```python
from build123d import *

# Parameters (mm, degrees)
SALIENTE_EXTRUIR1_DEPTH = 30
CROQUIS2_R              = 2.5
CORTAR_EXTRUIR1_DEPTH   = 71.10083252
CROQUIS3_W              = 27
CROQUIS3_H              = 62.627315121
CORTAR_EXTRUIR2_DEPTH   = 72
CORTAR_EXTRUIR3_DEPTH   = 64.283609709


with BuildPart() as part:
    # Croquis1 → Saliente-Extruir1 (new body)
    with BuildSketch(Plane.XY):
        with BuildLine():
            Line((-13.910195184, 10.658823529), (-13.910195184, 39.47248109))
            ThreePointArc((-13.910195184, 39.47248109), (-12.082079753, 42.831486511), (-8.268736475, 43.12016711))
            Line((-8.268736475, 43.12016711), (46.089804816, 18.658823529))
            Line((46.089804816, 18.658823529), (46.089804816, 10.658823529))
            Line((46.089804816, 10.658823529), (-13.910195184, 10.658823529))
        make_face()
    extrude(amount=SALIENTE_EXTRUIR1_DEPTH)

    # Croquis2 → Cortar-Extruir1 (cut, through all)
    with BuildSketch(Plane.XY.offset(30)):
        with Locations((-9.910195184, 39.47248109)):
            Circle(CROQUIS2_R)
    extrude(amount=-CORTAR_EXTRUIR1_DEPTH, mode=Mode.SUBTRACT)

    # Croquis3 → Cortar-Extruir2 (cut)
    with BuildSketch(Plane.ZY.offset(13.910195184)):
        with Locations((15, 43.47248109)):
            Rectangle(CROQUIS3_W, CROQUIS3_H)
    extrude(amount=-CORTAR_EXTRUIR2_DEPTH, mode=Mode.SUBTRACT)

    # Croquis4 → Cortar-Extruir3 (cut, through all)
    with BuildSketch(Plane(origin=(0, 12.158823529, 0), x_dir=(1, 0, 0), z_dir=(0, 1, 0))):
        with BuildLine():
            Line((-33.910195184, -20), (6.089804816, -20))
            ThreePointArc((6.089804816, -20), (11.089804816, -15), (6.089804816, -10))
            Line((6.089804816, -10), (-33.910195184, -10))
            Line((-33.910195184, -10), (-33.910195184, -20))
        make_face()
    extrude(amount=-CORTAR_EXTRUIR3_DEPTH, mode=Mode.SUBTRACT)


solid = part.part
```
Geometry: final body of the model. Coordinates: model frame, mm. A direction names the side the tool comes from. Round coordinates to 2 decimals unless told otherwise and drop trailing zeros. Loops run counter-clockwise (first coordinate to the right, second up) from the corner with the lowest first, then second, coordinate; pieces in that order, holes last. Notation, with made-up numbers: (35, -16) -> (83, -16) arc R17 cw to (83, 16) -> close; hole circle Ø10 at (65.5, 28.5). An arc over 180 degrees is marked (long way). Use one line per item in the form item = value.
Item 1: Material intervals for probe 1 along Z at (x, y) = (41, 14); probe 2 along Y at (x, z) = (31, 21.25), sorted ascending.
Evaluation:
probe_1 = 0 to 1.5, 28.5 to 30
probe_2 = 10.66 to 12.16
Item 2: Cut plane C-C on y = 38. Output: boundary loops of the cut face in (x, z), then the cut area to 3 significant figures.
Evaluation:
outline = (-13.91, 0) -> (-11.93, 0) -> (-11.93, 1.5) -> (-13.91, 1.5) -> close; (-13.91, 28.5) -> (-11.93, 28.5) -> (-11.93, 30) -> (-13.91, 30) -> close; (-7.89, 0) -> (3.11, 0) -> (3.11, 1.5) -> (-7.89, 1.5) -> close; (-7.89, 28.5) -> (3.11, 28.5) -> (3.11, 30) -> (-7.89, 30) -> close
area = 38.9 mm2
Item 3: Cut plane A-A on y = 17.5. Output: boundary loops of the cut face in (x, z), then the cut area to 3 significant figures.
Evaluation:
outline = (-13.91, 0) -> (46.09, 0) -> (46.09, 1.5) -> (-13.91, 1.5) -> close; (-13.91, 28.5) -> (46.09, 28.5) -> (46.09, 30) -> (-13.91, 30) -> close
area = 180 mm2
Item 4: Draft query along X for faces 4 (the cylindrical face through (11.09, 11.42, 15.11)), 5 (the cylindrical face through (-11.753, 41.162, 29.26)), 6 (the flat face through (46.09, 12, 18)), 7 (the cylindrical face through (-11.753, 41.162, 0.761)). Return one class per face: released by +X, released by -X, zero draft, split by the parting line, or undercut.
Evaluation:
face_4 = released by -X
face_5 = undercut
face_6 = released by +X
face_7 = undercut
Item 5: Cut plane D-D on x = 37. Output: boundary loops of the cut face in (y, z).
Evaluation:
outline = (10.66, 0) -> (22.75, 0) -> (22.75, 1.5) -> (12.16, 1.5) -> (12.16, 28.5) -> (22.75, 28.5) -> (22.75, 30) -> (10.66, 30) -> close
Item 6: Access query for faces 1 (the flat face through (-4, 11, 10)), 2 (the flat face through (18.53, 31.06, 29.24)), 3 (the flat face through (16, 12.159, 15)). Directions: +Z, -Z, +X, -X, +Y, -Y. A direction counts if a zero-diameter tool reaches every point of the face in a straight line with its end or side. Return the directions, or none.
Evaluation:
face_1 = -X, +Y, -Y
face_2 = +Z, -Z, +X, +Y
face_3 = +X, -X, +Y
Item 7: Cut plane B-B on x = -1. Output: boundary loops of the cut face in (y, z).
Evaluation:
outline = (10.66, 0) -> (39.85, 0) -> (39.85, 1.5) -> (12.16, 1.5) -> (12.16, 10) -> (10.66, 10) -> close; (10.66, 20) -> (12.16, 20) -> (12.16, 28.5) -> (39.85, 28.5) -> (39.85, 30) -> (10.66, 30) -> close
